from build123d import *

# Parameters (mm, degrees)
F0_W     = 68.5234218836
F0_H     = 74.8608410358
F1_DEPTH = 4
F2_R     = 2.63906
F3_DEPTH = 4.001
F4_W     = 1.2
F4_H     = 50.72188
F5_DEPTH = 4
F6_R     = 0.254
F7_R     = 12.7
F8_DEPTH = 38.1
F8_TAPER = 18


with BuildPart() as f1:
    # F0 (on Front) → F1 (new body)
    with BuildSketch(Plane.XZ):
        Rectangle(F0_W, F0_H)
    extrude(amount=F1_DEPTH)

    # F2 (on face) → F3 (cut, through all)
    with BuildSketch(Plane.XZ.offset(4)):
        with Locations((-34.2617109418, 28)):
            Circle(F2_R)
        with Locations((15.2382890582, 13.5)):
            Circle(F2_R)
        with Locations((-34.2617109418, -28)):
            Circle(F2_R)
        with Locations((15.2382890582, -13.5)):
            Circle(F2_R)
        with BuildLine():
            Line((20.95, 8.5), (7.6382890582, 8.5))
            Line((7.6382890582, 8.5), (7.6382890582, 0))
            Line((7.6382890582, 0), (34.2617109418, 0))
            Line((34.2617109418, 0), (34.2617109418, 8.5))
            Line((34.2617109418, 8.5), (34.2617109418, 37.4304205179))
            Line((34.2617109418, 37.4304205179), (-34.2617109418, 37.4304205179))
            Line((-34.2617109418, 37.4304205179), (-34.2617109418, 32.5))
            Line((-34.2617109418, 32.5), (0, 32.5))
            ThreePointArc((0, 32.5), (14.1412738111, 27.0425492812), (20.95, 13.5))
            Line((20.95, 13.5), (20.95, 8.5))
        make_face()
        with BuildLine():
            Line((34.2617109418, 0), (7.6382890582, 0))
            Line((7.6382890582, 0), (7.6382890582, -8.5))
            Line((7.6382890582, -8.5), (20.95, -8.5))
            Line((20.95, -8.5), (20.95, -13.5))
            ThreePointArc((20.95, -13.5), (14.1412738111, -27.0425492812), (0, -32.5))
            Line((0, -32.5), (-34.2617109418, -32.5))
            Line((-34.2617109418, -32.5), (-34.2617109418, -37.4304205179))
            Line((-34.2617109418, -37.4304205179), (34.2617109418, -37.4304205179))
            Line((34.2617109418, -37.4304205179), (34.2617109418, -8.5))
            Line((34.2617109418, -8.5), (34.2617109418, 0))
        make_face()
    extrude(amount=-F3_DEPTH, mode=Mode.SUBTRACT)

    # F4 (on face) → F5 (join, through all)
    with BuildSketch(Plane.XZ.offset(4)):
        with BuildLine():
            Line((-34.2617109418, -32.5), (-34.2617109418, -30.63906))
            Line((-34.2617109418, -30.63906), (-36.0617109418, -30.63906))
            ThreePointArc((-36.0617109418, -30.63906), (-37.3930806688, -31.1815330645), (-37.9662013504, -32.5))
            Line((-37.9662013504, -32.5), (-34.2617109418, -32.5))
        make_face()
        with Locations((-34.8617109418, 0)):
            Rectangle(F4_W, F4_H)
        with BuildLine():
            Line((-36.0617109418, 30.63906), (-34.2617109418, 30.63906))
            Line((-34.2617109418, 30.63906), (-34.2617109418, 32.5))
            Line((-34.2617109418, 32.5), (-37.9662013504, 32.5))
            ThreePointArc((-37.9662013504, 32.5), (-37.3930806688, 31.1815330645), (-36.0617109418, 30.63906))
        make_face()
    extrude(amount=-F5_DEPTH)

    # F6
    f6_edges = [f1.edges().sort_by_distance(p)[0] for p in [
        (-37.966201, -2, -32.5),
        (-37.966201, -2, 32.5),
    ]]
    fillet(f6_edges, radius=F6_R)

    # F7 (on face) → F8 (join)
    with BuildSketch(Plane.XZ.offset(4)):
        with Locations((-12.6483709418, 0)):
            Circle(F7_R)
    extrude(amount=F8_DEPTH, taper=F8_TAPER)


solid = f1.part
Verification items for the finished model (mm, model axes). A direction names the side the tool comes from. Coordinates: 2 decimals unless noted, no trailing zeros. Order: outer loops, then holes, each group sorted by start corner. A loop starts at its lowest first (then second) coordinate and runs counter-clockwise, first axis right, second up.
Item 1: Depth check by flat-ended pin: pin 1 (3 mm diameter, centred on y = -2.5, z = 0.5, fed in from +X); pin 2 (4.5 mm diameter, centred on y = -1.5, z = -1, fed in from -X); pin 3 (6 mm diameter, centred on x = -22, y = -9.5, fed in from +Z). Enter the tip coordinate at first touch or a pass-through.
Filled in:
pin 1: stops at x = 7.64
pin 2: stops at x = -35.46
pin 3: stops at z = 9.19
Item 2: Section check A-A, the plane z = 22.5. Enter the section's corners in (x, y), then the cut area to 3 significant figures.
Filled in:
outline: (-35.46, -4) - (17.92, -4) - (17.92, 0) - (-35.46, 0) - close
area: 214 mm2
Item 3: Section check B-B, the plane y = -18. Enter the section's corners in (x, z).
Filled in:
outline: circle Ø16.3 at (-12.65, 0)
Item 4: Access from +Z, -Z, +X, -X, +Y, -Y to the whole of each face (thin tool, end or side, straight path). Record for faces 1 (the face through (-17.38, -23.32, 4.34)), 2 (the face through (7.638, -2, 0)), 3 (the face through (-37.295, -2.028, 31.092)).
Filled in:
face 1: -Y
face 2: +X, +Y, -Y
face 3: -X, +Y, -Y
Item 5: Section check C-C, the plane z = -28. Enter the section's corners in (x, y), then the cut area to 3 significant figures.
Filled in:
outline: (-31.62, -4) - (13.01, -4) - (13.01, 0) - (-31.62, 0) - close
area: 179 mm2
Item 6: Material ranges on L1, parallel to Y at x = 7, z = 26; L2, parallel to Z at x = -14, y = -5.5; L3, parallel to X at y = -9, z = -7, recorded low to high.
Filled in:
L1: y = -4 to 0
L2: z = -12.14 to 12.14
L3: x = -21.23 to -4.07
Item 7: Release check for a two-part mould opening along X. For faces 4 (the face through (-37.27, -2.03, -31.07)), 5 (the face through (13.98, -2.028, 27.188)), 6 (the face through (12.6, -2, 13.6)) record: +X half, -X half, draft (parallel to the pull), parting line (faces both ways), or undercut.
Filled in:
face 4: -X half
face 5: +X half
face 6: undercut
